Read the model definition and answer for the solid it produces. Units are mm, in the model's axes. Round coordinates to 2 decimals unless told otherwise and drop trailing zeros. Loops run counter-clockwise (first coordinate to the right, second up) from the corner with the lowest first, then second, coordinate; pieces in that order, holes last. Notation, with made-up numbers: M 11,51.25 L 43,51.25 A6 cw 43,61.25 Z; hole C 28,72.5 d2. An arc over 180 degrees is marked long. Write each question's results on one line, items separated by ' | '.
from build123d import *

# Parameters (mm, degrees)
BOSS_EXTRUDE1_DEPTH = 1
SKETCH3_R           = 4
SKETCH3_R_2         = 2.5
CUT_EXTRUDE1_DEPTH  = 2


with BuildPart() as part:
    # Sketch2 → Boss-Extrude1 (new body)
    with BuildSketch(Plane.XY):
        Polygon((-20, 75.180318298), (20, 75.180318298), (30, -24.819681702), (-30, -24.819681702), align=None)
    extrude(amount=BOSS_EXTRUDE1_DEPTH)

    # Sketch3 → Cut-Extrude1 (cut, through all)
    with BuildSketch(Plane.XY.offset(1)):
        with Locations((18, -14.819681702)):
            Circle(SKETCH3_R)
        with Locations((-18, -14.819681702)):
            Circle(SKETCH3_R)
        with Locations((0, 60.180318298)):
            Circle(SKETCH3_R_2)
        with Locations((0, 30.180318298)):
            Circle(SKETCH3_R_2)
    extrude(amount=-CUT_EXTRUDE1_DEPTH, mode=Mode.SUBTRACT)


solid = part.part
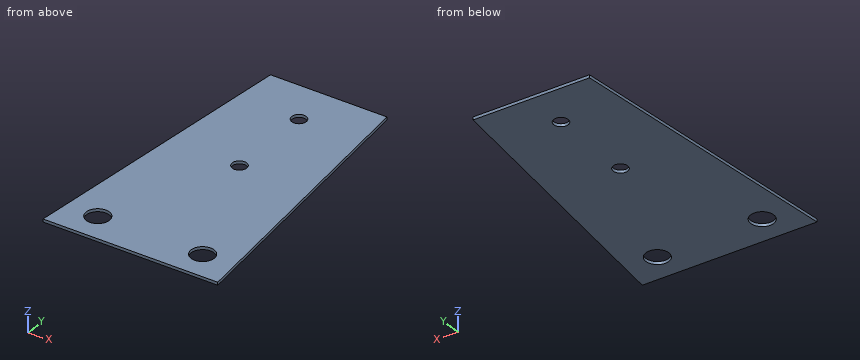
Item 1: Straight lines are drawn through the part: line 1 (Y direction, x = 0, z = 0.45); line 2 (Y direction, x = 18, z = 0.85); line 3 (Y direction, x = 1.5, z = 0.4). For each, find the intervals that lie inside material, in ascending order.
Outcome:
line 1: y = -24.82 to 27.68, 32.68 to 57.68, 62.68 to 75.18 | line 2: y = -24.82 to -18.82, -10.82 to 75.18 | line 3: y = -24.82 to 28.18, 32.18 to 58.18, 62.18 to 75.18
Item 2: The part is cut by section A-A (x = -18). Determine the outline of the cut face in (y, z), plus the area to 3 significant figures.
Outcome:
outline: M -24.82,0 L -18.82,0 L -18.82,1 L -24.82,1 Z; M -10.82,0 L 75.18,0 L 75.18,1 L -10.82,1 Z | area: 92.0 mm2
Item 3: A flat-ended cylindrical pin translates along its axis: pin 1 (4.5 mm diameter, centred on x = 0, y = 30.18, fed in from +Z). Find the tip coordinate at first contact, or state that the pin passes through.
Outcome:
pin 1: passes through
Item 4: The part is cut by section B-B (x = 0). Determine the outline of the cut face in (y, z), plus the area to 3 significant figures.
Outcome:
outline: M -24.82,0 L 27.68,0 L 27.68,1 L -24.82,1 Z; M 32.68,0 L 57.68,0 L 57.68,1 L 32.68,1 Z; M 62.68,0 L 75.18,0 L 75.18,1 L 62.68,1 Z | area: 90.0 mm2
Item 5: The part is cut by section C-C (z = 0.2). Determine the outline of the cut face in (x, y), plus the area to 3 significant figures.
Outcome:
outline: M -30,-24.82 L 30,-24.82 L 20,75.18 L -20,75.18 Z; hole C -18,-14.82 d8; hole C 0,30.18 d5; hole C 0,60.18 d5; hole C 18,-14.82 d8 | area: 4,860 mm2
Item 6: The part is cut by section D-D (y = 48.5). Determine the outline of the cut face in (x, z).
Outcome:
outline: M -22.67,0 L 22.67,0 L 22.67,1 L -22.67,1 Z
